The model under review builds one solid part; all positions refer to its coordinate system, in mm. A direction names the side the tool comes from. Round coordinates to 2 decimals unless told otherwise and drop trailing zeros. Order: outer loops, then holes, each group sorted by start corner. A loop starts at its lowest first (then second) coordinate and runs counter-clockwise, first axis right, second up. Notation, with made-up numbers: (2.25, 69.25) -> (36.25, 69.25) arc R34 ccw to (36.25, 108.25) -> close; hole circle Ø4 at (-36.75, 16.25). An arc over 180 degrees is marked (long way). Put each result on its own line as item: value. Start each with the question number.
from build123d import *

# Parameters (mm, degrees)
SKETCH_1_W          = 15
SKETCH_1_H          = 15
SKETCH_1_W_2        = 12
SKETCH_1_H_2        = 12
EXTRUDE_1_DEPTH     = 500
SKETCH_2_R          = 2.7
CUT_EXTRUDE_1_DEPTH = 25
SKETCH_3_R          = 2.25
CUT_EXTRUDE_2_DEPTH = 25
SKETCH_4_R          = 2.25
CUT_EXTRUDE_3_DEPTH = 20
SKETCH_5_R          = 5
CUT_EXTRUDE_4_DEPTH = 10
SKETCH_6_R          = 5
CUT_EXTRUDE_5_DEPTH = 10


with BuildPart() as part:
    # ｽｹｯﾁ1 → ﾎﾞｽ - 押し出し1 (new body)
    with BuildSketch(Plane.XY):
        Rectangle(SKETCH_1_W, SKETCH_1_H)
        Rectangle(SKETCH_1_W_2, SKETCH_1_H_2, mode=Mode.SUBTRACT)
    extrude(amount=EXTRUDE_1_DEPTH)

    # ｽｹｯﾁ2 → ｶｯﾄ - 押し出し1 (cut)
    with BuildSketch(Plane(origin=(7.5, 0, 0), x_dir=(0, 0, -1), z_dir=(1, 0, 0))):
        with Locations((-492.5, 0)):
            Circle(SKETCH_2_R)
        with Locations((-7.5, 0)):
            Circle(SKETCH_2_R)
        with Locations((-317.5, 0)):
            Circle(SKETCH_2_R)
        with Locations((-182.5, 0)):
            Circle(SKETCH_2_R)
    extrude(amount=-CUT_EXTRUDE_1_DEPTH, mode=Mode.SUBTRACT)

    # ｽｹｯﾁ3 → ｶｯﾄ - 押し出し2 (cut)
    with BuildSketch(Plane(origin=(0, 7.5, 0), x_dir=(1, 0, 0), z_dir=(0, 1, 0))):
        with Locations((0, -22.5)):
            Circle(SKETCH_3_R)
        with Locations((0, -477.5)):
            Circle(SKETCH_3_R)
    extrude(amount=-CUT_EXTRUDE_2_DEPTH, mode=Mode.SUBTRACT)

    # ｽｹｯﾁ4 → ｶｯﾄ - 押し出し3 (cut)
    with BuildSketch(Plane(origin=(0, -7.5, 0), x_dir=(-1, 0, 0), z_dir=(0, -1, 0))):
        with Locations((0, -390)):
            Circle(SKETCH_4_R)
        with Locations((0, -330)):
            Circle(SKETCH_4_R)
        with Locations((0, -110)):
            Circle(SKETCH_4_R)
        with Locations((0, -170)):
            Circle(SKETCH_4_R)
    extrude(amount=-CUT_EXTRUDE_3_DEPTH, mode=Mode.SUBTRACT)

    # ｽｹｯﾁ5 → ｶｯﾄ - 押し出し4 (cut)
    with BuildSketch(Plane(origin=(0, -7.5, 0), x_dir=(1, 0, 0), z_dir=(0, 1, 0))):
        with Locations((0, -22.5)):
            Circle(SKETCH_5_R)
        with Locations((0, -477.5)):
            Circle(SKETCH_5_R)
        with Locations((0, -390)):
            Circle(SKETCH_5_R)
        with Locations((0, -330)):
            Circle(SKETCH_5_R)
        with Locations((0, -110)):
            Circle(SKETCH_5_R)
        with Locations((0, -170)):
            Circle(SKETCH_5_R)
    extrude(amount=CUT_EXTRUDE_4_DEPTH, mode=Mode.SUBTRACT)

    # ｽｹｯﾁ6 → ｶｯﾄ - 押し出し5 (cut)
    with BuildSketch(Plane(origin=(7.5, 0, 0), x_dir=(0, 0, -1), z_dir=(1, 0, 0))):
        with Locations((-492.5, 0)):
            Circle(SKETCH_6_R)
        with Locations((-317.5, 0)):
            Circle(SKETCH_6_R)
        with Locations((-182.5, 0)):
            Circle(SKETCH_6_R)
        with Locations((-7.5, 0)):
            Circle(SKETCH_6_R)
    extrude(amount=-CUT_EXTRUDE_5_DEPTH, mode=Mode.SUBTRACT)


solid = part.part
Q1. Wall thickness on probe 1 along X at (y, z) = (-2.5, 458); probe 2 along Y at (x, z) = (6.7, 7.5): over which ranges is each line inside the solid? List them lowest first. Write a range as [from, to].
Q2. For faces 4 (the face through (-6, 0, 246)), 5 (the face through (-0.651, -6.76, 385.043)), 6 (the face through (6.76, 1.5, 312.73)), list the 3-axis set-ups (+Z, -Z, +X, -X, +Y, -Y) from which the entire face can be reached by the end or side of a thin tool; tool diameter is ignored.
Q3. Take a section at A-A on z = 88.5. Give the boundary of the cut face in (x, y), and give its area (3 significant figures).
Q4. Clearance check with flat-ended pins moving along their axes: pin 1 Ø8 at (x, z) = (0, 330) entering from -Y; pin 2 Ø6 at (x, y) = (-2, 0) entering from +Z. State where each tip first meets the part, or that it passes through.
Q5. Draft analysis for pull direction X (two halves, no side actions). For faces 1 (the face through (0, -6, 246)), 2 (the face through (-7, 0, 500)), 3 (the face through (-7.5, 0, 246)), state which applies: +X half, -X half, draft (parallel to the pull), parting line (faces both ways), or undercut.
Calculated:
1. probe 1: x = [-7.5, -6], [6, 7.5]
1. probe 2: y = [-7.5, -5], [5, 7.5]
2. face 4: +Z, -Z
2. face 5: -Y
2. face 6: +X
3. outline: (-7.5, -7.5) -> (7.5, -7.5) -> (7.5, 7.5) -> (-7.5, 7.5) -> close; hole (-6, -6) -> (6, -6) -> (6, 6) -> (-6, 6) -> close
3. area: 81.0 mm²
4. pin 1: stops at y = 6
4. pin 2: passes through
5. face 1: undercut
5. face 2: draft
5. face 3: -X half
